from build123d import *

# Parameters (mm, degrees)
F0_R     = 3.302
F0_R_2   = 12.5
F1_DEPTH = 3.048
F2_D     = 3.75
F3_R     = 5.08
F4_R     = 5.08


with BuildPart() as f1:
    # F0 (on Top) → F1 (new body)
    with BuildSketch(Plane.XY):
        with BuildLine():
            Line((-50.6614250383, 139.7), (-76.2, 139.7))
            Line((-76.2, 139.7), (-76.2, -139.7))
            Line((-76.2, -139.7), (76.2, -139.7))
            Line((76.2, -139.7), (76.2, 139.7))
            Line((76.2, 139.7), (50.6614250383, 139.7))
            ThreePointArc((50.6614250383, 139.7), (52.970732405, 135.8563312628), (53.775, 131.445))
            ThreePointArc((53.775, 131.445), (36.8636687372, 119.749267595), (31.8885749617, 139.7))
            Line((31.8885749617, 139.7), (-31.8885749617, 139.7))
            ThreePointArc((-31.8885749617, 139.7), (-29.579267595, 135.8563312628), (-28.775, 131.445))
            ThreePointArc((-28.775, 131.445), (-45.6863312628, 119.749267595), (-50.6614250383, 139.7))
        make_face()
        with BuildLine():
            ThreePointArc((-72.66317, -84.6626662669), (-70.78817, -82.7876662669), (-68.91317, -84.6626662669))
            Line((-68.91317, -84.6626662669), (-68.91317, -110.0626662669))
            ThreePointArc((-68.91317, -110.0626662669), (-70.78817, -111.9376662669), (-72.66317, -110.0626662669))
            Line((-72.66317, -110.0626662669), (-72.66317, -84.6626662669))
        make_face(mode=Mode.SUBTRACT)
        with BuildLine():
            ThreePointArc((-72.66317, -41.5120462669), (-70.78817, -39.6370462669), (-68.91317, -41.5120462669))
            Line((-68.91317, -41.5120462669), (-68.91317, -66.9120462669))
            ThreePointArc((-68.91317, -66.9120462669), (-70.78817, -68.7870462669), (-72.66317, -66.9120462669))
            Line((-72.66317, -66.9120462669), (-72.66317, -41.5120462669))
        make_face(mode=Mode.SUBTRACT)
        with BuildLine():
            ThreePointArc((-72.66317, 1.6385737331), (-70.78817, 3.5135737331), (-68.91317, 1.6385737331))
            Line((-68.91317, 1.6385737331), (-68.91317, -23.7614262669))
            ThreePointArc((-68.91317, -23.7614262669), (-70.78817, -25.6364262669), (-72.66317, -23.7614262669))
            Line((-72.66317, -23.7614262669), (-72.66317, 1.6385737331))
        make_face(mode=Mode.SUBTRACT)
        with Locations((0, -130.9944583397)):
            Circle(F0_R, mode=Mode.SUBTRACT)
        with BuildLine():
            ThreePointArc((67.975, -84.6626662669), (69.85, -82.7876662669), (71.725, -84.6626662669))
            Line((71.725, -84.6626662669), (71.725, -110.0626662669))
            ThreePointArc((71.725, -110.0626662669), (69.85, -111.9376662669), (67.975, -110.0626662669))
            Line((67.975, -110.0626662669), (67.975, -84.6626662669))
        make_face(mode=Mode.SUBTRACT)
        with BuildLine():
            ThreePointArc((67.975, -41.5120462669), (69.85, -39.6370462669), (71.725, -41.5120462669))
            Line((71.725, -41.5120462669), (71.725, -66.9120462669))
            ThreePointArc((71.725, -66.9120462669), (69.85, -68.7870462669), (67.975, -66.9120462669))
            Line((67.975, -66.9120462669), (67.975, -41.5120462669))
        make_face(mode=Mode.SUBTRACT)
        with BuildLine():
            ThreePointArc((67.975, 1.6385737331), (69.85, 3.5135737331), (71.725, 1.6385737331))
            Line((71.725, 1.6385737331), (71.725, -23.7614262669))
            ThreePointArc((71.725, -23.7614262669), (69.85, -25.6364262669), (67.975, -23.7614262669))
            Line((67.975, -23.7614262669), (67.975, 1.6385737331))
        make_face(mode=Mode.SUBTRACT)
        with BuildLine():
            ThreePointArc((-72.66317, 44.7891937331), (-70.78817, 46.6641937331), (-68.91317, 44.7891937331))
            Line((-68.91317, 44.7891937331), (-68.91317, 19.3891937331))
            ThreePointArc((-68.91317, 19.3891937331), (-70.78817, 17.5141937331), (-72.66317, 19.3891937331))
            Line((-72.66317, 19.3891937331), (-72.66317, 44.7891937331))
        make_face(mode=Mode.SUBTRACT)
        with BuildLine():
            ThreePointArc((-72.66317, 87.9398137331), (-70.78817, 89.8148137331), (-68.91317, 87.9398137331))
            Line((-68.91317, 87.9398137331), (-68.91317, 62.5398137331))
            ThreePointArc((-68.91317, 62.5398137331), (-70.78817, 60.6648137331), (-72.66317, 62.5398137331))
            Line((-72.66317, 62.5398137331), (-72.66317, 87.9398137331))
        make_face(mode=Mode.SUBTRACT)
        with Locations((-41.275, 76.835)):
            Circle(F0_R_2, mode=Mode.SUBTRACT)
        with BuildLine():
            ThreePointArc((67.975, 44.7891937331), (69.85, 46.6641937331), (71.725, 44.7891937331))
            Line((71.725, 44.7891937331), (71.725, 19.3891937331))
            ThreePointArc((71.725, 19.3891937331), (69.85, 17.5141937331), (67.975, 19.3891937331))
            Line((67.975, 19.3891937331), (67.975, 44.7891937331))
        make_face(mode=Mode.SUBTRACT)
        with Locations((41.275, 76.835)):
            Circle(F0_R_2, mode=Mode.SUBTRACT)
        with BuildLine():
            Line((67.975, 62.5398137331), (67.975, 87.9398137331))
            ThreePointArc((67.975, 87.9398137331), (69.85, 89.8148137331), (71.725, 87.9398137331))
            Line((71.725, 87.9398137331), (71.725, 62.5398137331))
            ThreePointArc((71.725, 62.5398137331), (69.85, 60.6648137331), (67.975, 62.5398137331))
        make_face(mode=Mode.SUBTRACT)
    extrude(amount=-F1_DEPTH)

    # F2 (through all)
    with Locations(Plane.XY):
        with Locations((-69.865, 101.6), (-55.865, 101.6), (27.9793004394, 45.5965413487), (27.9793004394, -44.5734586513), (55.865, 101.6), (69.865, 101.6), (22.5162935781, -68.6938670802), (22.5162935781, -109.3338670802), (63.1562935781, -109.3338670802), (63.1562935781, -68.6938670802), (-55.865, -128.4), (-69.865, -128.4), (55.865, -128.4), (69.865, -128.4), (0, 131.445), (0, 74.676), (-22.5, 129.7), (22.5, 129.7), (13.5, 2.7), (-13.5, 2.7)):
            Hole(F2_D / 2)

    # F3
    f3_edges = [f1.edges().sort_by_distance(p)[0] for p in [
        (-76.2, 139.7, -1.524),
        (76.2, 139.7, -1.524),
        (76.2, -139.7, -1.524),
        (-76.2, -139.7, -1.524),
    ]]
    fillet(f3_edges, radius=F3_R)

    # F4
    f4_edges = [f1.edges().sort_by_distance(p)[0] for p in [
        (-50.661425, 139.7, -1.524),
        (-31.888575, 139.7, -1.524),
        (31.888575, 139.7, -1.524),
        (50.661425, 139.7, -1.524),
    ]]
    fillet(f4_edges, radius=F4_R)


solid = f1.part
Could you check a few things on this model? Use its own coordinates, in mm. Give positions to 0.01 mm unless a question says otherwise; leave off trailing zeros. Order: outer loops, then holes, each group sorted by start corner. A loop starts at its lowest first (then second) coordinate and runs counter-clockwise, first axis right, second up.
1. Suppose I cut it at C-C (z = -1.25). Give the number of separate pieces and of enclosed holes in the cut face, plus the area to 3 significant figures.
2. Suppose I cut it at A-A (y = -57). List the corners of the cut face in (x, z) for me (3 decimals), plus the area to 3 significant figures.
3. Suppose I cut it at B-B (x = 45.5). List the corners of the cut face in (y, z) for me.
4. Will these pins go through, and if not, where does the flat tip stop? P1, Ø15, axis at x = 41.275, y = 76.835, coming from the +Z side; P2, Ø6, axis at x = -55.865, y = 101.6, coming from the +Z side.
5. I need wall thicknesses on L1, parallel to X at y = -6.5, z = -1.3 (3 decimals); L2, parallel to Y at x = 22.5, z = -1.7 (3 decimals); L3, parallel to Y at x = 13.5, z = -2.05 (3 decimals). Which ranges of each line are inside material? Lowest first, please.
6. We'd pull the mould along Y, two halves only. Please class faces 1 (the cylindrical face through (-0.43, -127.72, -1.5)), 2 (the flat face through (-1, 2, -3.048)), 3 (the cylindrical face through (-74.751, -138.172, -1.545)), 4 (the cylindrical face through (39.65, 89.23, -1.5)): pulls with the +Y half, pulls with the -Y half, needs draft (parallel to the pull), parting line crosses it, or undercut.
Solved:
1. separate pieces: 1
1. enclosed holes: 33
1. area: 39,300 mm2
2. outline: (-76.2, -3.048) - (-72.663, -3.048) - (-72.663, 0) - (-76.2, 0) - close; (-68.913, -3.048) - (67.975, -3.048) - (67.975, 0) - (-68.913, 0) - close; (71.725, -3.048) - (76.2, -3.048) - (76.2, 0) - (71.725, 0) - close
2. area: 442 mm2
3. outline: (-139.7, -3.05) - (65.07, -3.05) - (65.07, 0) - (-139.7, 0) - close; (88.6, -3.05) - (119.68, -3.05) - (119.68, 0) - (88.6, 0) - close
4. P1: passes through
4. P2: stops at z = 0
5. L1: x = -76.2 to -72.663, -68.913 to 67.975, 71.725 to 76.2
5. L2: y = -139.7 to -111.209, -107.459 to -70.569, -66.819 to 127.825, 131.575 to 139.7
5. L3: y = -139.7 to 0.825, 4.575 to 139.7
6. face 1: undercut
6. face 2: needs draft
6. face 3: pulls with the -Y half
6. face 4: undercut
